from build123d import *

# Parameters (mm, degrees)
F0_W     = 381
F0_H     = 12.7
F1_DEPTH = 539.75
F3_DEPTH = 654.05


with BuildPart() as f1:
    # F0 (on Right) → F1 (new body)
    with BuildSketch(Plane.YZ):
        with Locations((0, 635)):
            Rectangle(F0_W, F0_H)
    extrude(amount=F1_DEPTH)

    # F2 (on face) → F3 (join)
    with BuildSketch(Plane(origin=(0, 0, 628.65), x_dir=(1, 0, 0), z_dir=(0, 0, -1))):
        with BuildLine():
            Line((19.685, 187.325), (5.715, 187.325))
            ThreePointArc((5.715, 187.325), (3.918949, 186.581051), (3.175, 184.785))
            Line((3.175, 184.785), (3.175, 170.815))
            ThreePointArc((3.175, 170.815), (3.918949, 169.018949), (5.715, 168.275))
            Line((5.715, 168.275), (19.685, 168.275))
            ThreePointArc((19.685, 168.275), (21.481051, 169.018949), (22.225, 170.815))
            Line((22.225, 170.815), (22.225, 184.785))
            ThreePointArc((22.225, 184.785), (21.481051, 186.581051), (19.685, 187.325))
        make_face()
        with BuildLine():
            ThreePointArc((19.685, -187.325), (21.481051, -186.581051), (22.225, -184.785))
            Line((22.225, -184.785), (22.225, -170.815))
            ThreePointArc((22.225, -170.815), (21.481051, -169.018949), (19.685, -168.275))
            Line((19.685, -168.275), (5.715, -168.275))
            ThreePointArc((5.715, -168.275), (3.918949, -169.018949), (3.175, -170.815))
            Line((3.175, -170.815), (3.175, -184.785))
            ThreePointArc((3.175, -184.785), (3.918949, -186.581051), (5.715, -187.325))
            Line((5.715, -187.325), (19.685, -187.325))
        make_face()
    extrude(amount=F3_DEPTH)


solid = f1.part
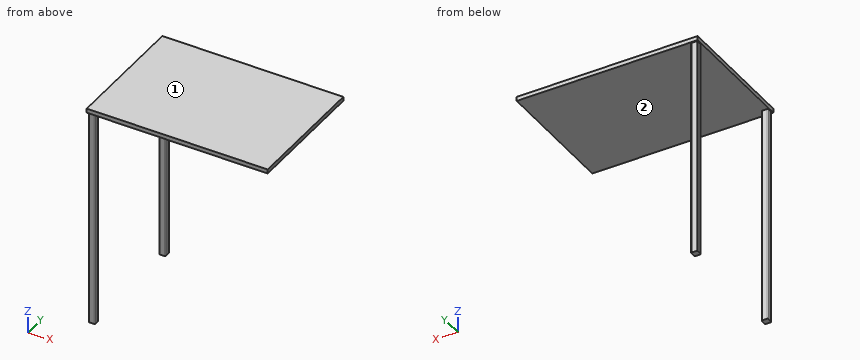
Design review of the part built by this model. Coordinates are the model's own, in mm. Face numbers are marked on the shaded views. Give positions to 0.01 mm unless a question says otherwise; leave off trailing zeros. Write each loop counter-clockwise with the first axis right and the second up, starting at its lowest first coordinate (ties: lowest second). Pieces come first, ordered by that corner, then holes. Notation, with made-up numbers: M 84,9.25 L 142,9.25 A17 ccw 142,37.25 Z; hole C -15.75,-32 d5. An arc over 180 degrees is marked long. Return JSON: item names as keys, results as strings. Group by question number.
Item 1: The part is to be moulded in two halves that separate along Z. For the marked faces 1 and 2, say which applies: pulls with the +Z half, pulls with the -Z half, needs draft (parallel to the pull), parting line crosses it, or undercut.
Item 2: Take a section at B-B (y = -13). Give the boundary of the cut face in (x, z), plus the area to 3 significant figures.
Item 3: Take a section at A-A (z = 231.5). Give the boundary of the cut face in (x, y) (3 decimals), plus the area to 3 significant figures.
Item 4: Clearance check with flat-ended pins moving along their axes: pin 1 Ø11 at (x, z) = (16, 210.5) entering from -Y (3 decimals); pin 2 Ø15.5 at (x, z) = (10, 167.5) entering from +Y (3 decimals); pin 3 Ø6 at (x, y) = (403.5, 76.5) entering from -Z. State where each tip first meets the part, or that it passes through.
Item 5: Take a section at C-C (x = 97.5). Give the boundary of the cut face in (y, z), plus the area to 3 significant figures.
Item 6: Wall thickness on line 1 along Z through (x, y) = (206, 15): over which ranges is the line inside the solid? List them lowest first.
Return value:
{
 "1": {"face 1": "pulls with the +Z half", "face 2": "pulls with the -Z half"},
 "2": {"outline": "M 0,628.65 L 539.75,628.65 L 539.75,641.35 L 0,641.35 Z", "area": "6,850 mm2"},
 "3": {"outline": "M 3.175,-184.785 A2.54 ccw 5.715,-187.325 L 19.685,-187.325 A2.54 ccw 22.225,-184.785 L 22.225,-170.815 A2.54 ccw 19.685,-168.275 L 5.715,-168.275 A2.54 ccw 3.175,-170.815 Z; M 3.175,170.815 A2.54 ccw 5.715,168.275 L 19.685,168.275 A2.54 ccw 22.225,170.815 L 22.225,184.785 A2.54 ccw 19.685,187.325 L 5.715,187.325 A2.54 ccw 3.175,184.785 Z", "area": "715 mm2"},
 "4": {"pin 1": "stops at y = -187.325", "pin 2": "stops at y = 187.325", "pin 3": "stops at z = 628.65"},
 "5": {"outline": "M -190.5,628.65 L 190.5,628.65 L 190.5,641.35 L -190.5,641.35 Z", "area": "4,840 mm2"},
 "6": {"line 1": "z = 628.65 to 641.35"}
}
